Autodesk Inventor part; units mm, degrees
ref_plane "YZ Plane" through (0, 0, 0) normal (1, 0, 0) x (0, 1, 0)
ref_plane "XZ Plane" through (0, 0, 0) normal (0, 1, 0) x (-1, 0, 0)
ref_plane "XY Plane" through (0, 0, 0) normal (0, 0, 1) x (1, 0, 0)
sketch "Sketch1" plane through (0, 0, 0) normal (1, 0, 0) x (0, 1, 0)
  line L0 (0, 0) -> (-30, 0)
  line L1 (-30, 0) -> (-30, -160)
  line L2 (-30, -160) -> (0, -160)
  line L3 (0, -160) -> (0, 0)
  circle A0 centre (-15, -14) radius 7.5
  circle A1 centre (-15, -146) radius 7.5
  dimension "d0" = 30
  dimension "d1" = 160
  dimension "d3" = 15
  dimension "d5" = 15
extrude "Extrusion1" add sketch "Sketch1" along normal blind 5
sketch "Sketch2" plane through (5, 0, 0) normal (1, 0, 0) x (0, 0, -1)
  circle A0 centre (14, -15) radius 7.5
  arc A1 (14, 0) -> (14, -30) centre (14, -15) ccw
  line L0 (0, -30) -> (160, -30)
  circle A2 centre (146, -15) radius 7.5
  arc A3 (146, -30) -> (146, 0) centre (146, -15) ccw
  line L1 (146, -30) -> (161, -30)
  line L2 (161, -30) -> (161, 0)
  line L3 (161, 0) -> (146, 0)
  line L4 (14, 0) -> (-1, 0)
  line L5 (-1, 0) -> (-1, -30)
  line L6 (-1, -30) -> (14, -30)
  point P0 (0, 0)
  point P1 (-1, -15)
  point P2 (161, -15)
extrude "Extrusion2" cut sketch "Sketch2" along normal blind 10 contours A3 L3 L2 | A3 L2 L1 L0 | A1 L0 L6 L5 | A1 L5 L4
fillet "Fillet1" radius 15 4 edges at (2.5, 0, 0) (2.5, -30, 0) (2.5, 0, -160) (2.5, -30, -160)
sketch "Sketch3" plane through (5, 0, 0) normal (1, 0, 0) x (0, 0, -1)
  point P0 (0, 0)
equation "\"BendRadius\" = Thickness"
equation "\"BendReliefWidth\" = Thickness"
equation "\"BendReliefDepth\" = 0.5 * Thickness"
equation "\"CornerReliefSize\" = 4 * Thickness"
equation "\"MinimumRemnant\" = 2 * Thickness"
equation "\"TransitionRadius\" = BendRadius"
equation "\"JacobiRadiusSize\" = BendRadius"
equation "\"GapSize\" = Thickness"
properties part number "Acoplador"
Source: CAD feature listing. Evaluate the final solid. Frame: model axes, mm. Give positions to 0.01 mm unless a question says otherwise; leave off trailing zeros. Order: outer loops, then holes, each group sorted by start corner. A loop starts at its lowest first (then second) coordinate and runs counter-clockwise, first axis right, second up. Notation, with made-up numbers: (87.25, -34) -> (133.25, -34) arc R18 ccw to (133.25, -10) -> close; hole circle Ø2 at (-22.75, 58.5). An arc over 180 degrees is marked (long way). Use a Markdown table: item, result.
1) Section query C-C, the plane y = -25.5. Return the cut outline in (x, z), then the cut area to 3 significant figures.
Answer list:
| item | result |
|---|---|
| outline | (0, -155.71) -> (5, -155.71) -> (5, -4.29) -> (0, -4.29) -> close |
| area | 757 mm² |
2) Section query A-A, the plane x = 3.7. Count the separate pieces of the cut face and the enclosed holes in it, then the cut area to 3 significant figures.
Answer list:
| item | result |
|---|---|
| separate pieces | 1 |
| enclosed holes | 2 |
| area | 4,250 mm² |
3) Ray query, line 1 along Z through (x, y) = (3.5, -15); line 2 along Z through (x, y) = (4.55, -10); line 3 along Y through (x, z) = (0.85, -143). Return the intervals inside material, ascending. Write a range as [from, to].
Answer list:
| item | result |
|---|---|
| line 1 | [-160, -153.5], [-138.5, -21.5], [-6.5, 0] |
| line 2 | [-159.14, -151.59], [-140.41, -19.59], [-8.41, -0.86] |
| line 3 | [-30, -21.87], [-8.13, 0] |
4) Mould query, pull axis Y, two halves, no side actions, for faces 1 (the cylindrical face through (2.54, -25.72, -155.49)), 2 (the cylindrical face through (2.465, -15.976, -153.436)), 3 (the cylindrical face through (2.465, -20.952, -9.436)), 4 (the flat face through (0, -15, -79)). Classes: +Y half, -Y half, draft (parallel to the pull), parting line (faces both ways), or undercut.
Answer list:
| item | result |
|---|---|
| face 1 | -Y half |
| face 2 | undercut |
| face 3 | undercut |
| face 4 | draft |
5) Contact query for flat-ended pins moving along their axis: P1, Ø3, axis at x = 3.5, y = -19, coming from the +Z side; P2, Ø1, axis at x = 4, y = -6.5, coming from the -Z side; P3, Ø12, axis at y = -15, z = -14, coming from the +X side. Output: stop coordinate, or through.
Answer list:
| item | result |
|---|---|
| P1 | z = -0.21 |
| P2 | z = -157.69 |
| P3 | through |
6) Section query B-B, the plane y = -2. Return the cut outline in (x, z).
Answer list:
| item | result |
|---|---|
| outline | (0, -152.48) -> (5, -152.48) -> (5, -7.52) -> (0, -7.52) -> close |
